The model under review builds one solid part; all positions refer to its coordinate system, in mm. Face numbers are marked on the shaded views. A direction names the side the tool comes from. Coordinates: 2 decimals unless noted, no trailing zeros. Write each loop counter-clockwise with the first axis right and the second up, starting at its lowest first coordinate (ties: lowest second). Pieces come first, ordered by that corner, then holes. Notation, with made-up numbers: (18.25, 33.5) - (72.25, 33.5) arc R9 ccw to (72.25, 50.5) - close; hole circle Ø9 at (54.25, -24.5). An arc over 180 degrees is marked (long way). Put each result on its own line as item: value.
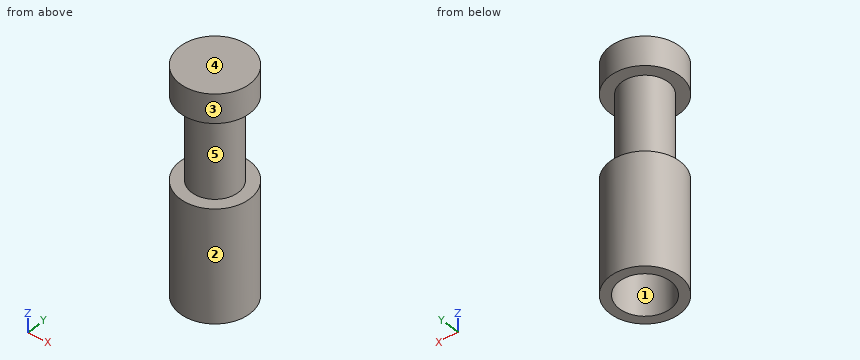
from build123d import *

# Parameters (mm, degrees)
SKETCH1_R           = 6
SKETCH1_R_2         = 4.4
BOSS_EXTRUDE1_DEPTH = 12
SKETCH2_R           = 6
BOSS_EXTRUDE2_DEPTH = 2
SKETCH3_R           = 4
BOSS_EXTRUDE3_DEPTH = 20
SKETCH4_R           = 6
BOSS_EXTRUDE4_DEPTH = 5
SKETCH5_R           = 6
BOSS_EXTRUDE5_DEPTH = 5.5


with BuildPart() as part:
    # Sketch1 → Boss-Extrude1 (new body)
    with BuildSketch(Plane.XY):
        Circle(SKETCH1_R)
        Circle(SKETCH1_R_2, mode=Mode.SUBTRACT)
    extrude(amount=BOSS_EXTRUDE1_DEPTH)

    # Sketch2 → Boss-Extrude2 (add)
    with BuildSketch(Plane.XY.offset(12)):
        Circle(SKETCH2_R)
    extrude(amount=BOSS_EXTRUDE2_DEPTH)

    # Sketch3 → Boss-Extrude3 (add)
    with BuildSketch(Plane.XY.offset(14)):
        Circle(SKETCH3_R)
    extrude(amount=BOSS_EXTRUDE3_DEPTH)

    # Sketch4 → Boss-Extrude4 (add)
    with BuildSketch(Plane.XY.offset(34)):
        Circle(SKETCH4_R)
    extrude(amount=BOSS_EXTRUDE4_DEPTH)

    # Sketch5 → Boss-Extrude5 (add)
    with BuildSketch(Plane.XY.offset(14)):
        Circle(SKETCH5_R)
    extrude(amount=BOSS_EXTRUDE5_DEPTH)


solid = part.part
1. Consider section C-C on z = 4.5. State the section outline as (x, y) points.
Determined:
outline: circle Ø12 at (0, 0); hole circle Ø8.8 at (0, 0)
2. Consider section A-A on x = 5.25. State the section outline as (y, z) points, plus the area to 3 significant figures.
Determined:
outline: (-2.9, 0) - (2.9, 0) - (2.9, 19.5) - (-2.9, 19.5) - close; (-2.9, 34) - (2.9, 34) - (2.9, 39) - (-2.9, 39) - close
area: 142 mm^2
3. Machinability: for the marked faces 1 and 2, which of the approach directions +Z, -Z, +X, -X, +Y, -Y give a long, thin tool a straight path to every point of the face, cutting with its end or side? Answer none if there is none.
Determined:
face 1: -Z
face 2: +Z, -Z
4. The part is to be moulded in two halves that separate along Z. For the marked faces 3, 4 and 5, say which applies: +Z half, -Z half, draft (parallel to the pull), parting line (faces both ways), or undercut.
Determined:
face 3: draft
face 4: +Z half
face 5: undercut
5. To check wall thickness, follow probe 1 along Z at (x, y) = (-4.5, -2); probe 2 along Y at (x, z) = (0, 6.25); probe 3 along Z at (x, y) = (-3.75, 2.25). State the ranges of each line that lie inside material, in increasing order.
Determined:
probe 1: z = 0 to 19.5, 34 to 39
probe 2: y = -6 to -4.4, 4.4 to 6
probe 3: z = 12 to 19.5, 34 to 39
6. For pin 1 Ø4 at (x, z) = (-4.5, 28.5) entering from +Y; pin 2 Ø6 at (y, z) = (-3, 21.5) entering from +X; pin 3 Ø1 at (x, y) = (1.5, 2) entering from -Z, all flat-tipped, find the tip position at first contact; note any pin that passes through.
Determined:
pin 1: stops at y = 3.12
pin 2: stops at x = 5.95
pin 3: stops at z = 12
7. Consider section B-B on x = 0. State the section outline as (y, z) points, plus the area to 3 significant figures.
Determined:
outline: (-6, 0) - (-4.4, 0) - (-4.4, 12) - (4.4, 12) - (4.4, 0) - (6, 0) - (6, 19.5) - (4, 19.5) - (4, 34) - (6, 34) - (6, 39) - (-6, 39) - (-6, 34) - (-4, 34) - (-4, 19.5) - (-6, 19.5) - close
area: 304 mm^2
